```python
from build123d import *

# Parameters (mm, degrees)
BOSS_EXTRUDE1_DEPTH     = 5
SKETCH2_R               = 0.25
CUT_EXTRUDE1_DEPTH      = 9
SKETCH4_R               = 0.25
CUT_EXTRUDE2_DEPTH      = 10
CUT_EXTRUDE2_DEPTH_BACK = 10


with BuildPart() as part:
    # Sketch1 → Boss-Extrude1 (new body)
    with BuildSketch(Plane.XY):
        Polygon((-6, 8), (-5, 8), (-5, 1), (5, 1), (5, 8), (6, 8), (6, 0), (-6, 0), align=None)
    extrude(amount=BOSS_EXTRUDE1_DEPTH)

    # Sketch2 → Cut-Extrude1 (cut, through all)
    with BuildSketch(Plane.XZ):
        with Locations((-5.5, 4.5)):
            Circle(SKETCH2_R)
        with Locations((-5.5, 0.5)):
            Circle(SKETCH2_R)
        with Locations((5.5, 4.5)):
            Circle(SKETCH2_R)
        with Locations((5.5, 0.5)):
            Circle(SKETCH2_R)
    extrude(amount=-CUT_EXTRUDE1_DEPTH, mode=Mode.SUBTRACT)

    # Sketch4 → Cut-Extrude2 (cut, two sides)
    with BuildSketch(Plane(origin=(0, 0, 0), x_dir=(0, 0, -1), z_dir=(1, 0, 0))) as cut_extrude2_sk:
        with Locations((-2.5, 4.5)):
            Circle(SKETCH4_R)
    extrude(amount=CUT_EXTRUDE2_DEPTH, mode=Mode.SUBTRACT)
    extrude(cut_extrude2_sk.sketch, amount=-CUT_EXTRUDE2_DEPTH_BACK, mode=Mode.SUBTRACT)


solid = part.part
```
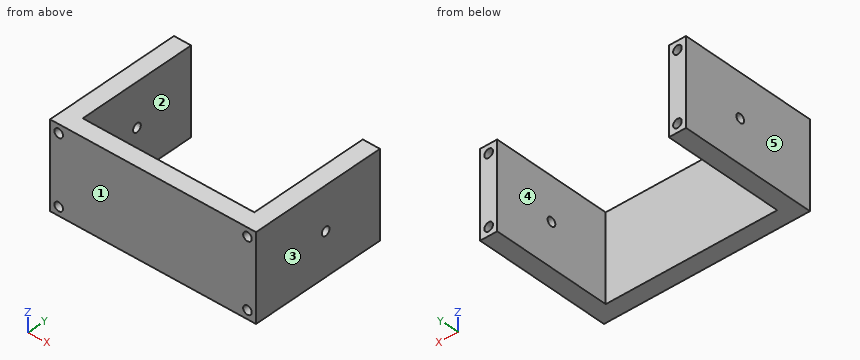
The model under review builds one solid part; all positions refer to its coordinate system, in mm. Face numbers are marked on the shaded views. A direction names the side the tool comes from. Coordinates: 2 decimals unless noted, no trailing zeros. Loops run counter-clockwise (first coordinate to the right, second up) from the corner with the lowest first, then second, coordinate; pieces in that order, holes last. Notation, with made-up numbers: (51.5, 15) -> (57.5, 15) arc R25 cw to (57.5, 43) -> close; hole circle Ø4 at (79.5, 60.5). An arc over 180 degrees is marked (long way). Answer as CSV lines item,"result".
Item 1: Take a section at D-D, the plane y = 4.5. State the section outline as (x, z) points.
Results below:
outline,"(-6, 0) -> (-5, 0) -> (-5, 2.25) -> (-6, 2.25) -> close; (-6, 2.75) -> (-5, 2.75) -> (-5, 5) -> (-6, 5) -> close; (5, 0) -> (6, 0) -> (6, 2.25) -> (5, 2.25) -> close; (5, 2.75) -> (6, 2.75) -> (6, 5) -> (5, 5) -> close; hole circle Ø0.5 at (-5.5, 0.5); hole circle Ø0.5 at (-5.5, 4.5); hole circle Ø0.5 at (5.5, 0.5); hole circle Ø0.5 at (5.5, 4.5)"
Item 2: Take a section at B-B, the plane x = -5.5. State the section outline as (y, z) points.
Results below:
outline,"(0, 0) -> (8, 0) -> (8, 0.25) -> (0, 0.25) -> close; (0, 0.75) -> (8, 0.75) -> (8, 4.25) -> (0, 4.25) -> close; (0, 4.75) -> (8, 4.75) -> (8, 5) -> (0, 5) -> close; hole circle Ø0.5 at (4.5, 2.5)"
Item 3: Insertion check: pin 1 (3 mm diameter, centred on x = 1.5, z = 1, fed in from +Y). The pin has a flat end and moves straight along its axis. Give the tip position at first contact, or say it passes through.
Results below:
pin 1,"stops at y = 1"
Item 4: Machinability: for the marked faces 4 and 5, which of the approach directions +Z, -Z, +X, -X, +Y, -Y give a long, thin tool a straight path to every point of the face, cutting with its end or side? Answer none if there is none.
Results below:
face 4,"+Z, -Z, +Y"
face 5,"+Z, -Z, -X, +Y, -Y"
Item 5: Draft analysis for pull direction X (two halves, no side actions). For the marked faces 1, 2 and 3, state which applies: +X half, -X half, draft (parallel to the pull), parting line (faces both ways), or undercut.
Results below:
face 1,"draft"
face 2,"undercut"
face 3,"+X half"
Item 6: Take a section at A-A, the plane y = 1.25. State the section outline as (x, z) points.
Results below:
outline,"(-6, 0) -> (-5, 0) -> (-5, 5) -> (-6, 5) -> close; (5, 0) -> (6, 0) -> (6, 5) -> (5, 5) -> close; hole circle Ø0.5 at (-5.5, 0.5); hole circle Ø0.5 at (-5.5, 4.5); hole circle Ø0.5 at (5.5, 0.5); hole circle Ø0.5 at (5.5, 4.5)"
Item 7: Take a section at C-C, the plane z = 4.5. State the section outline as (x, y) points.
Results below:
outline,"(-6, 0) -> (-5.75, 0) -> (-5.75, 8) -> (-6, 8) -> close; (-5.25, 0) -> (5.25, 0) -> (5.25, 8) -> (5, 8) -> (5, 1) -> (-5, 1) -> (-5, 8) -> (-5.25, 8) -> close; (5.75, 0) -> (6, 0) -> (6, 8) -> (5.75, 8) -> close"
Item 8: For L1, parallel to Z at x = 5.5, y = 4; L2, parallel to X at y = 1.25, z = 0.4; L3, parallel to Z at x = 5.45, y = 4.5, list the stretches that pass through material, from the lowest coordinate up.
Results below:
L1,"z = 0 to 0.25, 0.75 to 4.25, 4.75 to 5"
L2,"x = -6 to -5.73, -5.27 to -5, 5 to 5.27, 5.73 to 6"
L3,"z = 0 to 0.26, 0.74 to 2.25, 2.75 to 4.26, 4.74 to 5"
